Check sheet for the modelled part. Datum: model origin and axes. Units: mm. Face numbers are marked on the shaded views. Coordinates: 2 decimals unless noted, no trailing zeros. Loops run counter-clockwise (first coordinate to the right, second up) from the corner with the lowest first, then second, coordinate; pieces in that order, holes last. Notation, with made-up numbers: (88.5, 85) - (98.5, 85) arc R30 cw to (98.5, 110) - close; hole circle Ø2 at (42.5, -37). An arc over 180 degrees is marked (long way). Write each question's results on one line, items separated by ' | '. Start each with the question number.
1. Gauge pin test, flat ends, axial feed: P1, Ø5, axis at y = 3, z = 27.5, coming from the -X side; P2, Ø4, axis at y = -3, z = -15, coming from the -X side; P3, Ø5, axis at x = -12, y = 0, coming from the -Z side; P4, Ø2, axis at x = 0.5, y = -0.5, coming from the +Z side. Record the tip position at first contact, or that the pin passes through.
2. Draft check along Z on the marked faces 1, 2, 3 and 4. Enter one of: released by +Z, released by -Z, zero draft, split by the parting line, or undercut.
3. Cross-section at A-A (y = 0). Give the number of separate pieces and of enclosed holes in the cut face, and give its area (3 significant figures).
4. Cross-section at B-B (x = 12). Record the cut outline in (y, z), and give its area (3 significant figures).
5. Thickness scan on line 1 (Y direction, x = 20, z = 43); line 2 (Z direction, x = -1, y = -2.75); line 3 (X direction, y = -2.5, z = 9). Record the ranges inside material, lowest first. Write a range as [from, to].
6. Cross-section at C-C (z = -20). Record the cut outline in (x, y).
7. Cross-section at D-D (z = -1). Record the cut outline in (x, y).
```python
from build123d import *

# Parameters (mm, degrees)
F_3_8INCH_DEPTH    = 4.7625
SKETCH2_R          = 31.75
CUT_EXTRUDE1_DEPTH = 9.525
SKETCH3_R          = 2.2
M4_THROUGH_DEPTH   = 9.525
SKETCH4_R          = 2.15
M5X8_DRILL_DEPTH   = 8
SKETCH5_R          = 2.15
M5X8_DRILL2_DEPTH  = 8


with BuildPart() as part:
    # Sketch1 → 3/8inch (new, symmetric)
    with BuildSketch(Plane(origin=(0, 0, 0), x_dir=(1, 0, 0), z_dir=(0, 1, 0))):
        with BuildLine():
            Line((-30, -45), (30, -45))
            Line((30, -45), (40.997797218, -23.112824386))
            ThreePointArc((40.997797218, -23.112824386), (44.19360745, 15.165387766), (20, 45))
            Line((20, 45), (-20, 45))
            ThreePointArc((-20, 45), (-44.19360745, 15.165387766), (-40.997797218, -23.112824386))
            Line((-40.997797218, -23.112824386), (-30, -45))
        make_face()
    extrude(amount=F_3_8INCH_DEPTH, both=True)

    # Sketch2 → Cut-Extrude1 (cut)
    with BuildSketch(Plane(origin=(0, 4.7625, 0), x_dir=(1, 0, 0), z_dir=(0, 1, 0))):
        with Locations(Location((0, 0, 0), (0, 0, 270))):
            Circle(SKETCH2_R)
    extrude(amount=-CUT_EXTRUDE1_DEPTH, mode=Mode.SUBTRACT)

    # Sketch3 → M4_through (cut)
    with BuildSketch(Plane(origin=(0, 4.7625, 0), x_dir=(1, 0, 0), z_dir=(0, 1, 0))):
        with Locations(Location((17.75, 30.743901834, 0), (0, 0, 270))):
            Circle(SKETCH3_R)
        with Locations(Location((35.5, 0, 0), (0, 0, 270))):
            Circle(SKETCH3_R)
        with Locations(Location((17.75, -30.743901834, 0), (0, 0, 270))):
            Circle(SKETCH3_R)
        with Locations(Location((-17.75, -30.743901834, 0), (0, 0, 270))):
            Circle(SKETCH3_R)
        with Locations(Location((-35.5, 0, 0), (0, 0, 270))):
            Circle(SKETCH3_R)
        with Locations(Location((-17.75, 30.743901834, 0), (0, 0, 270))):
            Circle(SKETCH3_R)
    extrude(amount=-M4_THROUGH_DEPTH, mode=Mode.SUBTRACT)

    # Sketch4 → M5x8_DRILL (cut)
    with BuildSketch(Plane(origin=(0, 0, -45), x_dir=(-1, 0, 0), z_dir=(0, 0, -1))):
        with Locations((-12, 0)):
            Circle(SKETCH4_R)
        with Locations(Location((12, 0, 0), (0, 0, 180))):
            Circle(SKETCH4_R)
    extrude(amount=-M5X8_DRILL_DEPTH, mode=Mode.SUBTRACT)

    # Sketch5 → M5x8_DRILL2 (cut)
    with BuildSketch(Plane.XY.offset(45)):
        with Locations((-20, 0)):
            Circle(SKETCH5_R)
        with Locations(Location((20, 0, 0), (0, 0, 180))):
            Circle(SKETCH5_R)
        Circle(SKETCH5_R)
    extrude(amount=-M5X8_DRILL2_DEPTH, mode=Mode.SUBTRACT)


solid = part.part
```
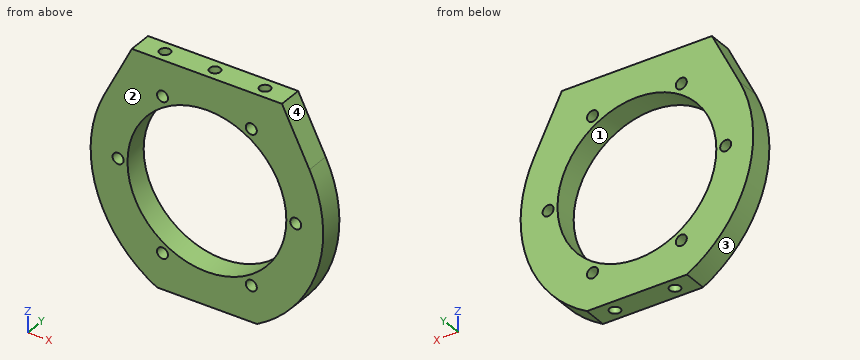
Established:
1) P1: x = -40.05 | P2: x = -44.81 | P3: z = -45 | P4: z = 37
2) face 1: undercut | face 2: zero draft | face 3: split by the parting line | face 4: released by +Z
3) separate pieces: 1 | enclosed holes: 7 | area: 3,680 mm^2
4) outline: (-4.76, -45) - (-2.15, -45) - (-2.15, -37) - (2.15, -37) - (2.15, -45) - (4.76, -45) - (4.76, -29.39) - (-4.76, -29.39) - close; (-4.76, 29.39) - (4.76, 29.39) - (4.76, 45) - (-4.76, 45) - close | area: 263 mm^2
5) line 1: [-4.76, -2.15], [2.15, 4.76] | line 2: [-45, -31.73], [31.73, 45] | line 3: [-45.69, -30.45], [30.45, 45.69]
6) outline: (-42.43, -4.76) - (-24.66, -4.76) - (-24.66, 4.76) - (-42.43, 4.76) - close; (24.66, -4.76) - (42.43, -4.76) - (42.43, 4.76) - (24.66, 4.76) - close
7) outline: (-46.47, -4.76) - (-37.46, -4.76) - (-37.46, 4.76) - (-46.47, 4.76) - close; (-33.54, -4.76) - (-31.73, -4.76) - (-31.73, 4.76) - (-33.54, 4.76) - close; (31.73, -4.76) - (33.54, -4.76) - (33.54, 4.76) - (31.73, 4.76) - close; (37.46, -4.76) - (46.47, -4.76) - (46.47, 4.76) - (37.46, 4.76) - close
